Geometry check sheet. Reference: the model listing, model coordinates, mm. A direction names the side the tool comes from. Coordinates: 2 decimals unless noted, no trailing zeros. Order: outer loops, then holes, each group sorted by start corner. A loop starts at its lowest first (then second) coordinate and runs counter-clockwise, first axis right, second up. Notation, with made-up numbers: (24.25, 31.25) - (64.25, 31.25) arc R24 ccw to (64.25, 46.25) - close; hole circle Ø3 at (-8, -1.5). An arc over 180 degrees is marked (long way). Return JSON: item names as keys, results as strings. Group by question number.
Item 1: Tool access check on faces 1 (the flat face through (-1, 45, 10)), 2 (the flat face through (-60, 39, 0)), 3 (the cylindrical face through (-45.636, 9.86, -59.517)). Record the directions out of +Z, -Z, +X, -X, +Y, -Y that give a thin tool (end or side, any length) a straight path to the whole face; none if there is none.
Item 2: Section check B-B on z = 0. Enter the section's corners in (x, y), then the cut area to 3 significant figures.
Item 3: Scan lines: probe 1 along Z at (x, y) = (46, 22.5); probe 2 along Y at (x, z) = (28, 24.5); probe 3 along Z at (x, y) = (-1, 9.5). Record each from-to range of solid material in increasing order.
Item 4: Section check D-D on y = 11.5. Enter the section's corners in (x, z), then the cut area to 3 significant figures.
Item 5: Section check A-A on x = 0. Enter the section's corners in (y, z).
Item 6: Section check C-C on y = 54. Enter the section's corners in (x, z), then the cut area to 3 significant figures.
Item 7: Gauge pin test, flat ends, axial feed: pin 1 (10 mm diameter, centred on y = 34, z = 4, fed in from +X); pin 2 (25 mm diameter, centred on x = 13, y = 46.5, fed in from +Z); pin 3 (1 mm diameter, centred on x = 3.5, z = 2.5, fed in from +Y). Record the tip position at first contact, or that the pin passes through.
Item 8: Draft check along Z on faces 4 (the flat face through (60, 39, 0)), 5 (the cylindrical face through (-1, 60, 0)), 6 (the flat face through (-1, 45, -10)). Enter one of: pulls with the +Z half, pulls with the -Z half, needs draft (parallel to the pull), parting line crosses it, or undercut.
from build123d import *

# Parameters (mm, degrees)
SKIZZE1_R                       = 75
AUFSATZ_LINEAR_AUSTRAGEN1_DEPTH = 20
SKIZZE2_W                       = 120
SKIZZE2_H                       = 20
AUFSATZ_LINEAR_AUSTRAGEN2_DEPTH = 50
SKIZZE4_R                       = 10
SCHNITT_LINEAR_AUSTRAGEN2_DEPTH = 122


with BuildPart() as part:
    # Skizze1 → Aufsatz-Linear austragen1 (new body)
    with BuildSketch(Plane(origin=(0, 0, 0), x_dir=(1, 0, 0), z_dir=(0, 1, 0))):
        with Locations(Location((0, 0, 0), (0, 0, 270))):
            Circle(SKIZZE1_R)
    extrude(amount=AUFSATZ_LINEAR_AUSTRAGEN1_DEPTH)

    # Skizze2 → Aufsatz-Linear austragen2 (add)
    with BuildSketch(Plane(origin=(0, 20, 0), x_dir=(1, 0, 0), z_dir=(0, 1, 0))):
        Rectangle(SKIZZE2_W, SKIZZE2_H)
    extrude(amount=AUFSATZ_LINEAR_AUSTRAGEN2_DEPTH)

    # Skizze4 → Schnitt-Linear austragen2 (cut)
    with BuildSketch(Plane.ZY.offset(60)):
        with Locations((0, 70)):
            Circle(SKIZZE4_R)
    extrude(amount=-SCHNITT_LINEAR_AUSTRAGEN2_DEPTH, mode=Mode.SUBTRACT)


solid = part.part
Computed:
{
 "1": {"face 1": "+Z, +X, -X, +Y", "face 2": "+Z, -Z, -X, +Y", "face 3": "+Y, -Y"},
 "2": {"outline": "(-75, 0) - (75, 0) - (75, 20) - (60, 20) - (60, 60) - (-60, 60) - (-60, 20) - (-75, 20) - close", "area": "7,800 mm²"},
 "3": {"probe 1": "z = -10 to 10", "probe 2": "y = 0 to 20", "probe 3": "z = -74.99 to 74.99"},
 "4": {"outline": "circle Ø150 at (0, 0)", "area": "17,700 mm²"},
 "5": {"outline": "(0, -75) - (20, -75) - (20, -10) - (70, -10) arc R10 cw to (70, 10) - (20, 10) - (20, 75) - (0, 75) - close"},
 "6": {"outline": "(-60, -10) - (60, -10) - (60, 10) - (-60, 10) - close", "area": "2,400 mm²"},
 "7": {"pin 1": "stops at x = 60", "pin 2": "stops at z = 10", "pin 3": "stops at y = 60.46"},
 "8": {"face 4": "needs draft", "face 5": "undercut", "face 6": "pulls with the -Z half"}
}
